The listing builds one solid part. Answer for the finished solid, in the listing's coordinates (mm). Give positions to 0.01 mm unless a question says otherwise; leave off trailing zeros. Order: outer loops, then holes, each group sorted by start corner. A loop starts at its lowest first (then second) coordinate and runs counter-clockwise, first axis right, second up. Notation, with made-up numbers: (51, -24) - (96, -24) arc R31 cw to (96, 6) - close; hole circle Ø3 at (78, 27.5). An arc over 180 degrees is marked (long way). Answer as a JSON object with one key per item and string values. Group by question number.
Q1. Consider line 1 (X direction, y = 13.5, z = -40); line 2 (Z direction, x = 125, y = 14.75); line 3 (Z direction, x = 560, y = 14). Determine where each line is inside the solid, lowest interval first.
Q2. The mould has two halves that part along Z. Classify faces 1 (the face through (554, 13, -25)), 2 (the face through (296, 13, 0)), 3 (the face through (296, 0, -64)): released by +Z, released by -Z, zero draft, split by the parting line, or undercut.
Q3. A cutting plane is placed at B-B, the plane z = -90. Give the vertices of the cut face in (x, y).
Q4. A cutting plane is placed at A-A, the plane x = 560. Give the vertices of the cut face in (y, z).
from build123d import *

# Parameters (mm, degrees)
SKETCH1_W           = 600
SKETCH1_H           = 127
BOSS_EXTRUDE1_DEPTH = 25.4
SKETCH2_R           = 6
CUT_EXTRUDE1_DEPTH  = 25.4
SKETCH3_R           = 5.25
CUT_EXTRUDE2_DEPTH  = 25.4


with BuildPart() as part:
    # Sketch1 → Boss-Extrude1 (new body)
    with BuildSketch(Plane(origin=(0, 0, 0), x_dir=(1, 0, 0), z_dir=(0, 1, 0))):
        with Locations((300, 63.5)):
            Rectangle(SKETCH1_W, SKETCH1_H)
    extrude(amount=BOSS_EXTRUDE1_DEPTH)

    # Sketch2 → Cut-Extrude1 (cut)
    with BuildSketch(Plane(origin=(0, 25.4, 0), x_dir=(1, 0, 0), z_dir=(0, 1, 0))):
        with Locations((40, 105)):
            Circle(SKETCH2_R)
        with Locations((40, 25)):
            Circle(SKETCH2_R)
        with Locations((560, 25)):
            Circle(SKETCH2_R)
        with Locations((560, 105)):
            Circle(SKETCH2_R)
    extrude(amount=-CUT_EXTRUDE1_DEPTH, mode=Mode.SUBTRACT)

    # Sketch3 → Cut-Extrude2 (cut)
    with BuildSketch(Plane(origin=(0, 25.4, 0), x_dir=(1, 0, 0), z_dir=(0, 1, 0))):
        with Locations((125, 90)):
            Circle(SKETCH3_R)
        with Locations((125, 40)):
            Circle(SKETCH3_R)
        with Locations((475, 40)):
            Circle(SKETCH3_R)
        with Locations((475, 90)):
            Circle(SKETCH3_R)
    extrude(amount=-CUT_EXTRUDE2_DEPTH, mode=Mode.SUBTRACT)


solid = part.part
Reply:
{
 "1": {"line 1": "x = 0 to 119.75, 130.25 to 469.75, 480.25 to 600", "line 2": "z = -127 to -95.25, -84.75 to -45.25, -34.75 to 0", "line 3": "z = -127 to -111, -99 to -31, -19 to 0"},
 "2": {"face 1": "undercut", "face 2": "released by +Z", "face 3": "zero draft"},
 "3": {"outline": "(0, 0) - (119.75, 0) - (119.75, 25.4) - (0, 25.4) - close; (130.25, 0) - (469.75, 0) - (469.75, 25.4) - (130.25, 25.4) - close; (480.25, 0) - (600, 0) - (600, 25.4) - (480.25, 25.4) - close"},
 "4": {"outline": "(0, -127) - (25.4, -127) - (25.4, -111) - (0, -111) - close; (0, -99) - (25.4, -99) - (25.4, -31) - (0, -31) - close; (0, -19) - (25.4, -19) - (25.4, 0) - (0, 0) - close"}
}
